Input: part model. Units: mm. Frame: model coordinates. Coordinates: 2 decimals unless noted, no trailing zeros. Loops run counter-clockwise (first coordinate to the right, second up) from the corner with the lowest first, then second, coordinate; pieces in that order, holes last. Notation, with made-up numbers: (3.25, -32) -> (38.25, -32) arc R25 ccw to (38.25, -17) -> close; hole circle Ø4 at (18.25, 41.25). An arc over 180 degrees is marked (long way). Put each result on its own line as item: value. Start each with the question number.
1) Contact query for flat-ended pins moving along their axis: P1, Ø1, axis at x = 21.5, y = -4.5, coming from the +Z side; P2, Ø2, axis at y = -5.5, z = 21, coming from the -X side; P3, Ø1.5, axis at x = -32, y = -1, coming from the +Z side; P4, Ø1.5, axis at x = 19, z = 34, coming from the -Y side. Output: stop coordinate, or through.
2) Cut plane B-B (x = -35). Return the cut outline in (y, z), plus the area to 3 significant figures.
3) Cut plane A-A (y = -1). Return the cut outline in (x, z).
4) Material intervals for L1, parallel to Z at x = -23, y = -4.5; L2, parallel to X at y = -1.75, z = 28; L3, parallel to Z at x = 11, y = -3.75, sorted ascending.
5) Cut plane C-C (z = 43.5). Return the cut outline in (x, y), plus the area to 3 significant figures.
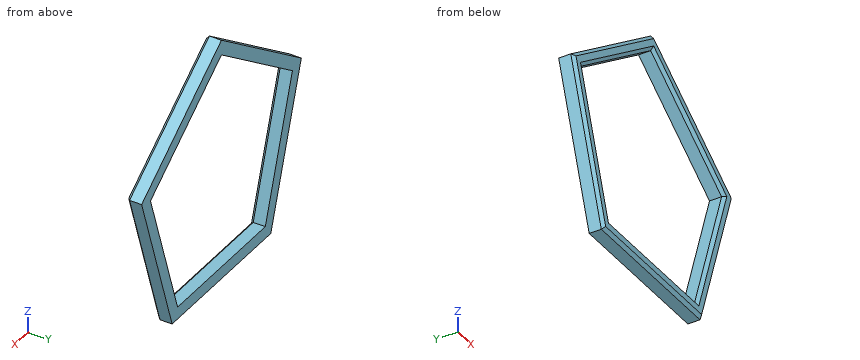
from build123d import *

# Parameters (mm, degrees)
F1_DEPTH = 6.35
F2_SIZE2 = 1.27
F2_SIZE  = 1.27


with BuildPart() as f1:
    # F0 (on Front) → F1 (new body)
    with BuildSketch(Plane.XZ):
        Polygon((54.35288, 17.660321), (0, 57.15), (-54.35288, 17.660321), (-33.591927, -46.235321), (33.591927, -46.235321), align=None)
        Polygon((-48.313671, 15.698063), (0, 50.8), (48.313671, 15.698063), (29.859491, -41.098063), (-29.859491, -41.098063), align=None, mode=Mode.SUBTRACT)
    extrude(amount=F1_DEPTH)

    # F2
    f2_edges = [f1.edges().sort_by_distance(p)[0] for p in [
        (43.972404, -6.35, -14.2875),
        (27.17644, -6.35, 37.405161),
        (-27.17644, -6.35, 37.405161),
        (-43.972404, -6.35, -14.2875),
        (0, -6.35, -46.235321),
        (-24.156836, -6.35, 33.249032),
        (24.156836, -6.35, 33.249032),
        (39.086581, -6.35, -12.7),
        (0, -6.35, -41.098063),
        (-39.086581, -6.35, -12.7),
    ]]
    chamfer(f2_edges, length=F2_SIZE, length2=F2_SIZE2)


solid = f1.part
Results found:
1. P1: stops at z = 41.89
1. P2: stops at x = -51.01
1. P3: stops at z = 34.45
1. P4: passes through
2. outline: (-6.35, -37.79) -> (-5.08, -41.9) -> (0, -41.9) -> (0, -25.28) -> (-5.08, -25.28) -> (-6.35, -29.39) -> close; (-6.35, 26.94) -> (-5.08, 25.37) -> (0, 25.37) -> (0, 31.72) -> (-5.08, 31.72) -> (-6.35, 30.15) -> close
2. area: 139 mm2
3. outline: (-54.35, 17.66) -> (-33.59, -46.24) -> (33.59, -46.24) -> (54.35, 17.66) -> (0, 57.15) -> close; hole (-48.31, 15.7) -> (-29.86, -41.1) -> (29.86, -41.1) -> (48.31, 15.7) -> (0, 50.8) -> close
4. L1: z = -46.24 to -41.1, 34.09 to 40.44
4. L2: x = -40.12 to -31.38, 31.38 to 40.12
4. L3: z = -46.24 to -41.1, 42.81 to 49.16
5. outline: (-18.79, -5.08) -> (-16.63, -6.35) -> (-12.21, -6.35) -> (-10.05, -5.08) -> (-10.05, 0) -> (-18.79, 0) -> close; (10.05, -5.08) -> (12.21, -6.35) -> (16.63, -6.35) -> (18.79, -5.08) -> (18.79, 0) -> (10.05, 0) -> close
5. area: 106 mm2
